```python
from build123d import *

# Parameters (mm, degrees)
F1_DEPTH = 8
F2_R     = 2.975
F3_DEPTH = 14


with BuildPart() as f1:
    # F0 (on Front) → F1 (new body)
    with BuildSketch(Plane.XZ):
        with BuildLine():
            Line((-15, 4.8), (-27.077851, 4.8))
            ThreePointArc((-27.077851, 4.8), (-27.5, 0), (-27.077851, -4.8))
            Line((-27.077851, -4.8), (-15, -4.8))
            ThreePointArc((-15, -4.8), (-10.2, 0), (-15, 4.8))
        make_face()
    extrude(amount=F1_DEPTH)

    # F2 (on face) → F3 (join)
    with BuildSketch(Plane(origin=(0, 0, 0), x_dir=(-1, 0, 0), z_dir=(0, 1, 0))):
        with Locations((20.077851, 0)):
            Circle(F2_R)
    extrude(amount=F3_DEPTH)


solid = f1.part
```
Build history of the part. All positions in model axes, mm. Round coordinates to 2 decimals unless told otherwise and drop trailing zeros. Loops run counter-clockwise (first coordinate to the right, second up) from the corner with the lowest first, then second, coordinate; pieces in that order, holes last. Notation, with made-up numbers: M 25.5,-26.5 L 72.5,-26.5 A22 cw 72.5,-3.5 Z; hole C 57,88 d5. An arc over 180 degrees is marked long. Answer as CSV lines item,"result".
1. Cut at B-B on x = -21.5. Write the cut outline in (y, z).
Resolved:
outline,"M -8,-4.8 L 0,-4.8 L 0,-2.61 L 14,-2.61 L 14,2.61 L 0,2.61 L 0,4.8 L -8,4.8 Z"
2. Two-plate mould, pull along Z, no slides. Class faces 1 (the flat face through (-20, 14, 0)), 2 (the flat face through (-21, -4, -4.8)), 3 (the cylindrical face through (-17.106, 6.902, 0.131)), 4 (the flat face through (-21, -4, 4.8)): released by +Z, released by -Z, zero draft, split by the parting line, or undercut.
Resolved:
face 1,"zero draft"
face 2,"released by -Z"
face 3,"split by the parting line"
face 4,"released by +Z"
3. Flat gauge pins, fed straight in: P1, Ø2, axis at y = 10, z = -1.5, coming from the -X side; P2, Ø1.5, axis at y = -0.5, z = -3.5, coming from the +X side; P3, Ø4, axis at x = -13, z = -1.5, coming from the +Y side. Where does each tip first touch, or does it go through?
Resolved:
P1,"stops at x = -23.01"
P2,"stops at x = -11.07"
P3,"stops at y = 0"
4. Wall check: probe 1 along Y at (x, z) = (-15.75, -4); probe 2 along X at (y, z) = (-2, -0.25); probe 3 along X at (y, z) = (9.75, -1.25). Give the ranges that are in metal, low to high. Write a range as [from, to].
Resolved:
probe 1,"y = [-8, 0]"
probe 2,"x = [-27.5, -10.21]"
probe 3,"x = [-22.78, -17.38]"
5. Cut at A-A on z = 0. Write the cut outline in (x, y), then the cut area to 3 significant figures.
Resolved:
outline,"M -27.5,-8 L -10.2,-8 L -10.2,0 L -17.1,0 L -17.1,14 L -23.05,14 L -23.05,0 L -27.5,0 Z"
area,"222 mm²"
6. Cut at C-C on y = -4. Write the cut outline in (x, z).
Resolved:
outline,"M -27.08,-4.8 L -15,-4.8 A4.8 ccw -15,4.8 L -27.08,4.8 A27.5 ccw Z"
7. Cut at D-D on x = -24.25. Write the cut outline in (y, z).
Resolved:
outline,"M -8,-4.8 L 0,-4.8 L 0,4.8 L -8,4.8 Z"
